The listing builds one solid part. Answer for the finished solid, in the listing's coordinates (mm). A direction names the side the tool comes from. Coordinates: 2 decimals unless noted, no trailing zeros. Order: outer loops, then holes, each group sorted by start corner. A loop starts at its lowest first (then second) coordinate and runs counter-clockwise, first axis right, second up. Notation, with made-up numbers: (27, 13) -> (79, 13) arc R36 cw to (79, 48) -> close; hole circle Ø7 at (-23, 18). An arc over 180 degrees is marked (long way). One line per question, with ' | ' between items.
from build123d import *

# Parameters (mm, degrees)
F0_W    = 0.75
F0_H    = 2.1
F0_W_2  = 1
F0_H_2  = 3.7
F2_SIZE = 0.2


with BuildPart() as f1:
    # F0 (on Front) → F1 (revolve)
    with BuildSketch(Plane.XZ):
        with Locations((-0.375, 2.25)):
            Rectangle(F0_W, F0_H)
        Polygon((-1.25, 1.2), (-1.25, 0), (-1, 0), (0, 0), (0, 1.2), (-0.75, 1.2), align=None)
        with Locations((-0.5, -1.85)):
            Rectangle(F0_W_2, F0_H_2)
        Polygon((0, -3.7), (-1, -3.7), (-0.930158, -5.7), (0, -5.7), align=None)
    revolve(axis=Axis((0, 0, -1.2), (0, 0, -1)))

    # F2
    f2_edges = [f1.edges().sort_by_distance(p)[0] for p in [
        (0.930158, 0, -5.7),
    ]]
    chamfer(f2_edges, length=F2_SIZE)


solid = f1.part
Item 1: This flat-tipped pin is pushed along its axis until it touches: pin 1 Ø1.5 at (y, z) = (0, -4.5) entering from -X. Where does it stop, or does it pass through?
Computed values:
pin 1: stops at x = -1
Item 2: Find the intervals of material crossed by L1, parallel to Z at x = -1.1, y = 0.3; L2, parallel to X at y = 0.55, z = -5; L3, parallel to Y at x = 0.65, z = -2.5, in increasing order.
Computed values:
L1: z = 0 to 1.2 | L2: x = -0.78 to 0.78 | L3: y = -0.76 to 0.76
Item 3: Section D-D, the plane z = -0.25 is taken. Give the vertices of the cut face in (x, y), plus the area to 3 significant figures.
Computed values:
outline: circle Ø2 at (0, 0) | area: 3.14 mm^2
Item 4: Section C-C, the plane z = 1 is taken. Give the vertices of the cut face in (x, y).
Computed values:
outline: circle Ø2.5 at (0, 0)
Item 5: For faces 1 (the face through (0, 0, 3.3)), 2 (the face through (0, -1, -2)), 3 (the face through (1, 0, 1.2)), determine the directions among +Z, -Z, +X, -X, +Y, -Y from which every point of the face is accessible in a straight line to the end or side of a thin tool.
Computed values:
face 1: +Z, +X, -X, +Y, -Y | face 2: -Z | face 3: +Z
Item 6: Section A-A, the plane y = 0 is taken. Give the vertices of the cut face in (x, z).
Computed values:
outline: (-1.25, 0) -> (-1, 0) -> (-1, -3.7) -> (-0.94, -5.5) -> (-0.73, -5.7) -> (0.73, -5.7) -> (0.94, -5.5) -> (1, -3.7) -> (1, 0) -> (1.25, 0) -> (1.25, 1.2) -> (0.75, 1.2) -> (0.75, 3.3) -> (-0.75, 3.3) -> (-0.75, 1.2) -> (-1.25, 1.2) -> close
